The listing builds one solid part. Answer for the finished solid, in the listing's coordinates (mm). Face numbers are marked on the shaded views. A direction names the side the tool comes from. Give positions to 0.01 mm unless a question says otherwise; leave off trailing zeros. Order: outer loops, then holes, each group sorted by start corner. A loop starts at its lowest first (then second) coordinate and runs counter-clockwise, first axis right, second up. Notation, with made-up numbers: M -22.75,79 L 4.25,79 A17 ccw 4.25,84 Z; hole C 63.5,83.5 d1. An arc over 180 degrees is marked long. Answer as a JSON object with one key per item and string values. Group by question number.
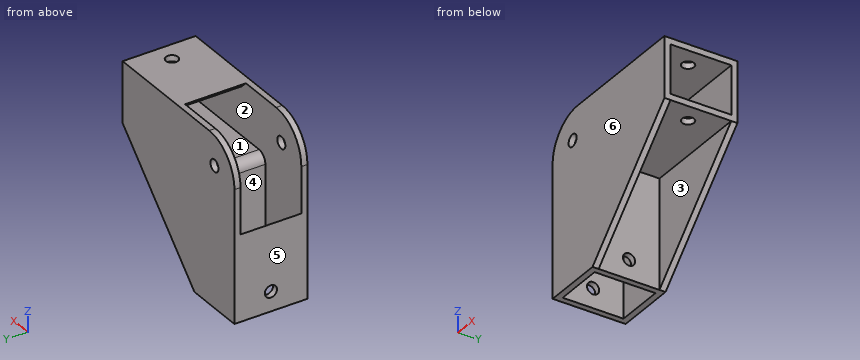
```python
from build123d import *

# Parameters (mm, degrees)
BOSS_EXTRUDE1_DEPTH     = 38.1
SKETCH2_W               = 25.4
SKETCH2_H               = 31.75
CUT_EXTRUDE1_DEPTH      = 88.9
CUT_EXTRUDE2_REACH      = 133.37
SKETCH3_W               = 25.4
SKETCH3_H               = 31.75
CUT_EXTRUDE3_START      = -62.861793
SKETCH4_W               = 75
SKETCH4_H               = 31.75
CUT_EXTRUDE3_DEPTH      = 28.575
FILLET4_R               = 20
CUT_EXTRUDE8_DEPTH      = 131.484388453
CUT_EXTRUDE8_DEPTH_BACK = 131.484388453
SKETCH8_R               = 3.175
BOSS_EXTRUDE2_DEPTH     = 3.175
CUT_EXTRUDE10_REACH     = 133.37
SKETCH35_R              = 3.175
CUT_EXTRUDE11_REACH     = 133.37
SKETCH36_R              = 3.175
FILLET8_R               = 5
CHAMFER1_SIZE           = 10
CHAMFER1_SIZE_2         = 7.071067812


with BuildPart() as part:
    # Sketch1 → Boss-Extrude1 (new body)
    with BuildSketch(Plane(origin=(0, 0, 0), x_dir=(1, 0, 0), z_dir=(0, 1, 0))):
        Polygon((0, 0), (-88.9, 0), (-88.9, 88.9), (-57.15, 88.9), (-57.15, 31.75), (0, 31.75), align=None)
    extrude(amount=BOSS_EXTRUDE1_DEPTH)

    # Sketch2 → Cut-Extrude1 (cut)
    with BuildSketch(Plane(origin=(0, 0, 0), x_dir=(0, 0, -1), z_dir=(1, 0, 0))):
        with Locations((15.875, 19.05)):
            Rectangle(SKETCH2_W, SKETCH2_H)
    extrude(amount=-CUT_EXTRUDE1_DEPTH, mode=Mode.SUBTRACT)

    # Cut-Extrude2: up to this face of the body (flat: up to its plane)
    cut_extrude2_end = Plane(part.part.faces().sort_by_distance((-44.45, 19.05, 0))[0])
    # Sketch3 → Cut-Extrude2 (cut, up to the picked face)
    with BuildSketch(Plane(origin=(0, 0, -88.9), x_dir=(-1, 0, 0), z_dir=(0, 0, -1)), mode=Mode.PRIVATE) as cut_extrude2_sk1:
        with Locations((73.025, 19.05)):
            Rectangle(SKETCH3_W, SKETCH3_H)
    cut_extrude2_tool1 = split(extrude(cut_extrude2_sk1.sketch, amount=-CUT_EXTRUDE2_REACH, mode=Mode.PRIVATE), bisect_by=cut_extrude2_end, keep=Keep.BOTH, mode=Mode.PRIVATE)
    add(cut_extrude2_tool1.solids().sort_by(Axis((-73.025, 19.05, -88.9), (0, 0, 1)))[0], mode=Mode.SUBTRACT)

    # Sketch4 → Cut-Extrude3 (cut)
    with BuildSketch(Plane(origin=(0, 0, 0), x_dir=(-0.7071067811865475, 0, -0.7071067811865476), z_dir=(0.7071067811865476, 0, -0.7071067811865475)).offset(CUT_EXTRUDE3_START)):
        with Locations((62.861792847, 19.05)):
            Rectangle(SKETCH4_W, SKETCH4_H)
    extrude(amount=CUT_EXTRUDE3_DEPTH, mode=Mode.SUBTRACT)

    # Fillet4
    fillet4_edges = [part.edges().sort_by_distance(p)[0] for p in [
        (-88.9, 36.5125, 0),
        (-88.9, 1.5875, 0),
    ]]
    fillet(fillet4_edges, radius=FILLET4_R)

    # Sketch8 → Cut-Extrude8 (cut, two sides: drawn at the far end of the back side and taken through both)
    with BuildSketch(Plane.XZ.offset(-34.925).offset(-CUT_EXTRUDE8_DEPTH_BACK)):
        with Locations(Location((-73.025, -15.875, 0), (0, 0, 270))):
            Circle(SKETCH8_R)
    extrude(amount=CUT_EXTRUDE8_DEPTH + CUT_EXTRUDE8_DEPTH_BACK, mode=Mode.SUBTRACT)

    # Sketch29 → Boss-Extrude2 (add)
    with BuildSketch(Plane(origin=(0, 38.1, 0), x_dir=(1, 0, 0), z_dir=(0, 1, 0))):
        Polygon((-57.15, 88.9), (0, 31.75), (-57.15, 31.75), align=None)
    boss_extrude2 = extrude(amount=-BOSS_EXTRUDE2_DEPTH)

    # Cut-Extrude10: up to this face of the body (flat: up to its plane)
    cut_extrude10_end = Plane(part.part.faces().sort_by_distance((-57.15, 17.4625, -60.325))[0])
    # Sketch35 → Cut-Extrude10 (cut, up to the picked face)
    with BuildSketch(Plane.ZY.offset(88.9), mode=Mode.PRIVATE) as cut_extrude10_sk1:
        with Locations((-78.65, 19.05)):
            Circle(SKETCH35_R)
    cut_extrude10_tool1 = split(extrude(cut_extrude10_sk1.sketch, amount=-CUT_EXTRUDE10_REACH, mode=Mode.PRIVATE), bisect_by=cut_extrude10_end, keep=Keep.BOTH, mode=Mode.PRIVATE)
    add(cut_extrude10_tool1.solids().sort_by(Axis((-88.9, 19.05, -78.65), (1, 0, 0)))[0], mode=Mode.SUBTRACT)

    # Cut-Extrude11: up to this face of the body (flat: up to its plane)
    cut_extrude11_end = Plane(part.part.faces().sort_by_distance((-28.575, 17.4625, -31.75))[0])
    # Sketch36 → Cut-Extrude11 (cut, up to the picked face)
    with BuildSketch(Plane.XY, mode=Mode.PRIVATE) as cut_extrude11_sk1:
        with Locations((-10.25, 19.05)):
            Circle(SKETCH36_R)
    cut_extrude11_tool1 = split(extrude(cut_extrude11_sk1.sketch, amount=-CUT_EXTRUDE11_REACH, mode=Mode.PRIVATE), bisect_by=cut_extrude11_end, keep=Keep.BOTH, mode=Mode.PRIVATE)
    add(cut_extrude11_tool1.solids().sort_by(Axis((-10.25, 19.05, 0), (0, 0, -1)))[0], mode=Mode.SUBTRACT)

    # Mirror1: Boss-Extrude2 across plane
    add(boss_extrude2.mirror(Plane(origin=(0, 19.05, 0), x_dir=(0, 0, 1), z_dir=(0, -1, 0))))

    # Fillet8
    fillet8_edges = [part.edges().sort_by_distance(p)[0] for p in [
        (-60.325, 19.05, -28.575),
    ]]
    fillet(fillet8_edges, radius=FILLET8_R)

    # Chamfer1
    # the kernel refuses this chamfer: 10, 7.071067812 mm, written as the material it takes off along each edge
    with BuildSketch(Plane(origin=(-51.663847671, 3.175, -3.175), x_dir=(0.9996219169112968, 0, -0.027495876610586317), z_dir=(0, 1, 0)), Plane(origin=(-85.725, 34.925, -37.236152329), x_dir=(0.027495876610586317, 0, -0.9996219169112968), z_dir=(0, -1, 0))) as chamfer1_piece_1:
        Polygon((CHAMFER1_SIZE * 0.999621916911, -CHAMFER1_SIZE * 0.0274958766106), (CHAMFER1_SIZE_2 * 0.687396915252, -CHAMFER1_SIZE_2 * 0.726281956863), (0, 0), align=None)
    extrude(amount=31.75, mode=Mode.SUBTRACT)


solid = part.part
```
Item 1: A tool of negligible diameter and unlimited length cuts with its end or side. For the marked faces 1, 2 and 3, from which of +Z, -Z, +X, -X, +Y, -Y can it reach the whole face along a straight path? Write none if from no direction.
Item 2: Flat-ended cylindrical pins translate along their axes: P1, Ø5.5, axis at y = 19.05, z = -78.65, coming from the +X side; P2, Ø7.5, axis at y = 19.05, z = -78.65, coming from the +X side; P3, Ø16, axis at x = -27.5, y = 26, coming from the -Z side. Find the tip coordinate at first contact, or state that the pin passes through.
Item 3: Section B-B (y = 13) is taken. Determine the outline of the cut face in (x, z) (3 decimals).
Item 4: Determine the mould class of the marked faces 4, 5 and 6 for opening direction Y: released by +Y, released by -Y, zero draft, split by the parting line, or undercut.
Item 5: Section D-D (z = -78.65) is taken. Determine the outline of the cut face in (x, y) (3 decimals), and give its area (3 significant figures).
Item 6: Section C-C (z = -51) is taken. Determine the outline of the cut face in (x, y) (3 decimals), and give its area (3 significant figures).
Item 7: Consider probe 1 along Y at (x, z) = (-34.5, -47) (3 decimals); probe 2 along Z at (x, y) = (-37, 34) (3 decimals); probe 3 along X at (y, z) = (4, -70) (3 decimals). Determine where each line is inside the solid, lowest interval first. Write a range as from..to.
Item 8: Section A-A (x = -10.25) is taken. Determine the outline of the cut face in (y, z) (3 decimals), and give its area (3 significant figures).
Values found:
{
 "1": {"face 1": "+X, -X", "face 2": "none", "face 3": "-Z, +X"},
 "2": {"P1": "passes through", "P2": "stops at x = -57.15", "P3": "stops at z = -31.75"},
 "3": {"outline": "M -88.9,-88.9 L -85.725,-88.9 L -85.725,-47.236 L -88.9,-44.061 Z; M -60.325,-88.9 L -57.15,-88.9 L -57.15,-31.75 L 0,-31.75 L 0,-28.575 L -55.325,-28.575 A5 ccw -60.325,-33.575 Z; M -44.839,0 L -41.664,-3.175 L 0,-3.175 L 0,0 Z"},
 "4": {"face 4": "undercut", "face 5": "zero draft", "face 6": "released by -Y"},
 "5": {"outline": "M -88.9,0 L -46.9,0 L -46.9,3.175 L -57.15,3.175 L -57.15,15.875 L -60.325,15.875 L -60.325,3.175 L -85.725,3.175 L -85.725,15.875 L -88.9,15.875 Z; M -88.9,22.225 L -85.725,22.225 L -85.725,34.925 L -60.325,34.925 L -60.325,22.225 L -57.15,22.225 L -57.15,34.925 L -46.9,34.925 L -46.9,38.1 L -88.9,38.1 Z", "area": "428 mm^2"},
 "6": {"outline": "M -88.9,0 L -19.25,0 L -19.25,3.175 L -57.15,3.175 L -57.15,34.925 L -19.25,34.925 L -19.25,38.1 L -88.9,38.1 Z; hole M -85.725,3.175 L -60.325,3.175 L -60.325,34.925 L -85.725,34.925 Z", "area": "644 mm^2"},
 "7": {"probe 1": "y = 0..3.175, 34.925..38.1", "probe 2": "z = -31.75..-28.575, -3.175..0", "probe 3": "x = -88.9..-85.725, -60.325..-57.15"},
 "8": {"outline": "M 0,-42 L 3.175,-42 L 3.175,-31.75 L 15.875,-31.75 L 15.875,-28.575 L 3.175,-28.575 L 3.175,-3.175 L 15.875,-3.175 L 15.875,0 L 0,0 Z; M 22.225,-31.75 L 34.925,-31.75 L 34.925,-42 L 38.1,-42 L 38.1,0 L 22.225,0 L 22.225,-3.175 L 34.925,-3.175 L 34.925,-28.575 L 22.225,-28.575 Z", "area": "428 mm^2"}
}
